Could you check a few things on this model? Use its own coordinates, in mm. Round coordinates to 2 decimals unless told otherwise and drop trailing zeros. Loops run counter-clockwise (first coordinate to the right, second up) from the corner with the lowest first, then second, coordinate; pieces in that order, holes last. Notation, with made-up numbers: (11, 35) -> (22, 35) arc R20 ccw to (22, 50) -> close; hole circle Ø3 at (-11.75, -27.75). An arc over 180 degrees is marked (long way). One line per item, written item: value.
Solid Edge part; units mm, degrees
sketch "Sketch1" plane through (0, 0, 0) normal (0, 0, 1) x (1, 0, 0)
  circle A0 centre (60, 240) radius 8.5
  line L0 (120, 280) -> (120, 0)
  line L1 (120, 0) -> (0, 0)
  line L2 (0, 0) -> (0, 280)
  arc A1 (10, 290) -> (0, 280) centre (10, 280) ccw
  line L3 (10, 290) -> (110, 290)
  arc A2 (120, 280) -> (110, 290) centre (110, 280) ccw
  circle A3 centre (60, 100) radius 8.5
extrude "Protrusion1" add sketch "Sketch1" along normal blind 4
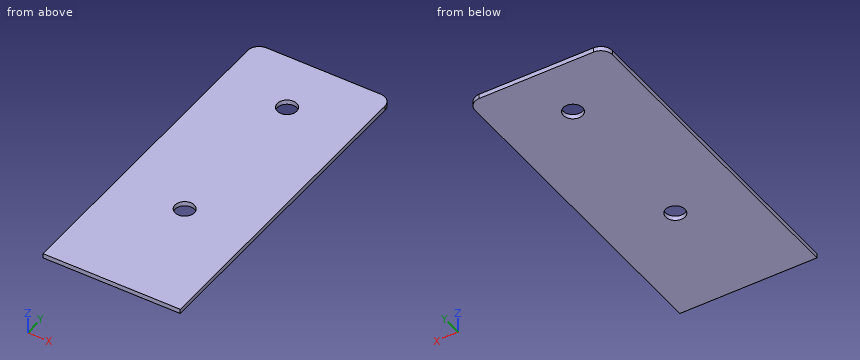
(1) If I drill on L1, parallel to Y at x = 59, z = 2.1; L2, parallel to Y at x = 60, z = 1.15; L3, parallel to Y at x = 5.5, z = 3.35, over which ranges is the centre line in solid material (lowest first)?
Recorded:
L1: 0 to 91.56, 108.44 to 231.56, 248.44 to 290
L2: 0 to 91.5, 108.5 to 231.5, 248.5 to 290
L3: 0 to 288.93
(2) If we section it at B-B, the plane y = 100: Please give me the cut outline in (x, z).
Recorded:
outline: (0, 0) -> (51.5, 0) -> (51.5, 4) -> (0, 4) -> close; (68.5, 0) -> (120, 0) -> (120, 4) -> (68.5, 4) -> close
(3) If we section it at A-A, the plane x = 60: Please give me the cut outline in (y, z), then the cut area to 3 significant figures.
Recorded:
outline: (0, 0) -> (91.5, 0) -> (91.5, 4) -> (0, 4) -> close; (108.5, 0) -> (231.5, 0) -> (231.5, 4) -> (108.5, 4) -> close; (248.5, 0) -> (290, 0) -> (290, 4) -> (248.5, 4) -> close
area: 1,020 mm²
